For this review, take the finished solid that the model builds, in its own axes (mm). Face numbers are marked on the shaded views. A direction names the side the tool comes from. Round coordinates to 2 decimals unless told otherwise and drop trailing zeros. Loops run counter-clockwise (first coordinate to the right, second up) from the corner with the lowest first, then second, coordinate; pieces in that order, holes last. Notation, with made-up numbers: M -19.75,6 L 21.25,6 A9 cw 21.25,19 Z; hole C -23,22.25 d5. An arc over 180 degrees is marked long. One line per question, with ' | ' between items. Start each with the question number.
1) We need section A-A (y = 13). Give the boundary of the cut face in (x, z), and give its area (3 significant figures).
2) For the marked faces 1, 2 and 3, list the 3-axis set-ups (+Z, -Z, +X, -X, +Y, -Y) from which the entire face can be reached by the end or side of a thin tool; tool diameter is ignored.
3) For pin 1 Ø11 at (x, y) = (72, 13.5) entering from +Z; pin 2 Ø1.5 at (x, z) = (70.5, 1.5) entering from +Y; pin 3 Ø4 at (y, z) = (4.5, 73.5) entering from +X, all flat-tipped, find the tip position at first contact; note any pin that passes through.
4) We need section B-B (z = 42.5). Give the boundary of the cut face in (x, y).
5) For probe 1 along Y at (x, z) = (-5, 75); probe 2 along Z at (x, y) = (0, 10.5); probe 3 along X at (y, z) = (9, 75), list the stretches that pass through material, from the lowest coordinate up. Write a range as from..to.
6) We need section C-C (x = 0). Give the boundary of the cut face in (y, z), and give its area (3 significant figures).
7) Mouldability with a two-part tool opening along Y and no side actions: class the marked faces 4, 5 and 6 as pulls with the +Y half, pulls with the -Y half, needs draft (parallel to the pull), parting line crosses it, or undercut.
8) We need section D-D (x = -47). Give the boundary of the cut face in (y, z), and give its area (3 significant figures).
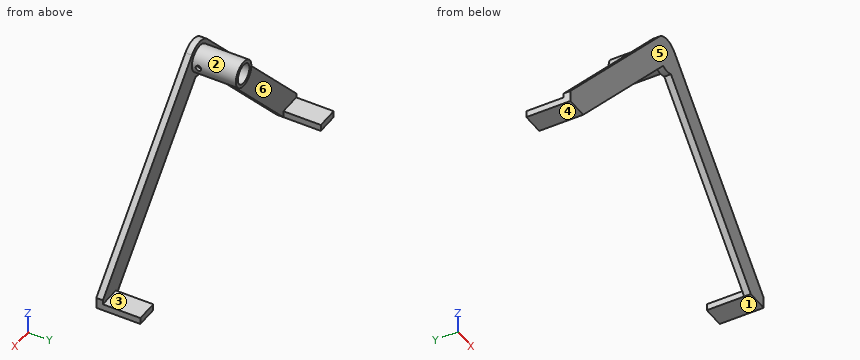
```python
from build123d import *

# Parameters (mm, degrees)
F1_DEPTH = 3
F2_R     = 6
F2_R_2   = 4.5
F3_DEPTH = 20
F4_W     = 10
F4_H     = 3
F5_DEPTH = 17
F6_R     = 1.25
F7_DEPTH = 12.5


with BuildPart() as f1:
    # F0 (on Front) → F1 (new body)
    with BuildSketch(Plane.XZ):
        with BuildLine():
            Line((-75, 5), (-75, 0))
            Line((-75, 0), (-65, 0))
            Line((-65, 0), (-3.0475954437, 67.6032330027))
            ThreePointArc((-3.0475954437, 67.6032330027), (0, 67), (3.0475954437, 67.6032330027))
            Line((3.0475954437, 67.6032330027), (65, 0))
            Line((65, 0), (75, 0))
            Line((75, 0), (75, 5))
            Line((75, 5), (5.8979816495, 80.4049803387))
            ThreePointArc((5.8979816495, 80.4049803387), (0, 83), (-5.8979816495, 80.4049803387))
            Line((-5.8979816495, 80.4049803387), (-75, 5))
        make_face()
    extrude(amount=-F1_DEPTH)

    # F2 (on face) → F3 (join)
    with BuildSketch(Plane(origin=(0, 3, 0), x_dir=(-1, 0, 0), z_dir=(0, 1, 0))):
        with Locations((0, 75)):
            Circle(F2_R)
        with Locations((0, 75)):
            Circle(F2_R_2, mode=Mode.SUBTRACT)
    extrude(amount=F3_DEPTH)

    # F4 (on face) → F5 (join)
    with BuildSketch(Plane(origin=(0, 3, 0), x_dir=(-1, 0, 0), z_dir=(0, 1, 0))):
        with Locations((-70, 1.5)):
            Rectangle(F4_W, F4_H)
        with Locations((70, 1.5)):
            Rectangle(F4_W, F4_H)
    extrude(amount=F5_DEPTH)

    # F6 (on Right) → F7 (cut, symmetric)
    with BuildSketch(Plane.YZ):
        with Locations((6, 75)):
            Circle(F6_R)
    extrude(amount=F7_DEPTH, both=True, mode=Mode.SUBTRACT)


solid = f1.part
```
Answers below:
1) outline: M -75,0 L -65,0 L -65,3 L -75,3 Z; C 0,75 d12; M 65,0 L 75,0 L 75,3 L 65,3 Z; hole C 0,75 d9 | area: 109 mm^2
2) face 1: -Z, +X, -X, +Y, -Y | face 2: +Y | face 3: +Z, +X, -X, +Y
3) pin 1: z = 3 | pin 2: y = 20 | pin 3: x = 13.44
4) outline: M -40.63,0 L -26.05,0 L -26.05,3 L -40.63,3 Z; M 26.05,0 L 40.63,0 L 40.63,3 L 26.05,3 Z
5) probe 1: 0..4.75, 7.25..23 | probe 2: 69..70.5, 79.5..81 | probe 3: -6..-4.5, 4.5..6
6) outline: M 0,67 L 3,67 L 3,69 L 23,69 L 23,70.5 L 3,70.5 L 3,79.5 L 23,79.5 L 23,81 L 3,81 L 3,83 L 0,83 Z | area: 108 mm^2
7) face 4: needs draft | face 5: pulls with the -Y half | face 6: pulls with the +Y half
8) outline: M 0,19.64 L 3,19.64 L 3,35.55 L 0,35.55 Z | area: 47.7 mm^2
